Input: part model. Units: mm. Frame: model coordinates. Face numbers are marked on the shaded views. Coordinates: 2 decimals unless noted, no trailing zeros. Order: outer loops, then holes, each group sorted by start corner. A loop starts at its lowest first (then second) coordinate and runs counter-clockwise, first axis right, second up. Notation, with made-up numbers: (38, -7.75) -> (54, -7.75) arc R23 ccw to (54, 16.25) -> close; hole circle Ø1 at (-6.5, -9.75). An arc over 180 degrees is marked (long way). Answer as CSV lines item,"result".
from build123d import *

# Parameters (mm, degrees)
F0_R     = 507.5
F0_R_2   = 16.5
F0_R_3   = 410
F1_DEPTH = 56


with BuildPart() as f1:
    # F0 (on Top) → F1 (new body)
    with BuildSketch(Plane.XY):
        Circle(F0_R)
        with Locations((-335.875721, -335.875721)):
            Circle(F0_R_2, mode=Mode.SUBTRACT)
        with Locations((-237.5, -411.362067)):
            Circle(F0_R_2, mode=Mode.SUBTRACT)
        with Locations((-122.939046, -458.814767)):
            Circle(F0_R_2, mode=Mode.SUBTRACT)
        with Locations((0, -475)):
            Circle(F0_R_2, mode=Mode.SUBTRACT)
        with Locations((-411.362067, -237.5)):
            Circle(F0_R_2, mode=Mode.SUBTRACT)
        with Locations((-458.814767, -122.939046)):
            Circle(F0_R_2, mode=Mode.SUBTRACT)
        with Locations((-475, 0)):
            Circle(F0_R_2, mode=Mode.SUBTRACT)
        Circle(F0_R_3, mode=Mode.SUBTRACT)
        with Locations((122.939046, -458.814767)):
            Circle(F0_R_2, mode=Mode.SUBTRACT)
        with Locations((237.5, -411.362067)):
            Circle(F0_R_2, mode=Mode.SUBTRACT)
        with Locations((335.875721, -335.875721)):
            Circle(F0_R_2, mode=Mode.SUBTRACT)
        with Locations((411.362067, -237.5)):
            Circle(F0_R_2, mode=Mode.SUBTRACT)
        with Locations((458.814767, -122.939046)):
            Circle(F0_R_2, mode=Mode.SUBTRACT)
        with Locations((475, 0)):
            Circle(F0_R_2, mode=Mode.SUBTRACT)
        with Locations((-458.814767, 122.939046)):
            Circle(F0_R_2, mode=Mode.SUBTRACT)
        with Locations((-411.362067, 237.5)):
            Circle(F0_R_2, mode=Mode.SUBTRACT)
        with Locations((-335.875721, 335.875721)):
            Circle(F0_R_2, mode=Mode.SUBTRACT)
        with Locations((-237.5, 411.362067)):
            Circle(F0_R_2, mode=Mode.SUBTRACT)
        with Locations((-122.939046, 458.814767)):
            Circle(F0_R_2, mode=Mode.SUBTRACT)
        with Locations((0, 475)):
            Circle(F0_R_2, mode=Mode.SUBTRACT)
        with Locations((458.814767, 122.939046)):
            Circle(F0_R_2, mode=Mode.SUBTRACT)
        with Locations((411.362067, 237.5)):
            Circle(F0_R_2, mode=Mode.SUBTRACT)
        with Locations((122.939046, 458.814767)):
            Circle(F0_R_2, mode=Mode.SUBTRACT)
        with Locations((237.5, 411.362067)):
            Circle(F0_R_2, mode=Mode.SUBTRACT)
        with Locations((335.875721, 335.875721)):
            Circle(F0_R_2, mode=Mode.SUBTRACT)
    extrude(amount=F1_DEPTH)


solid = f1.part
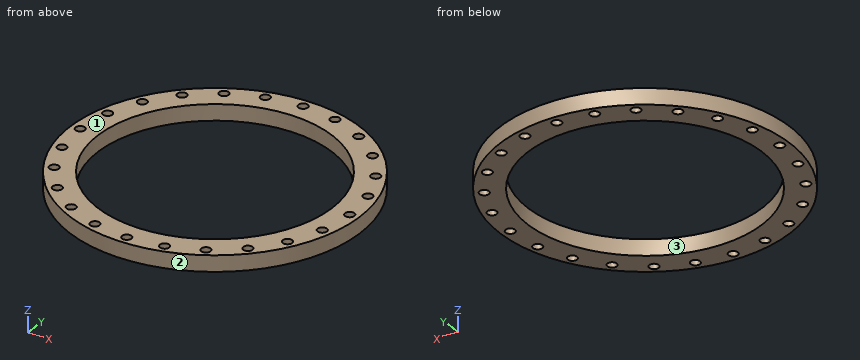
1. Cut plane A-A (y = 0). Return the cut outline in (x, z), plus the area to 3 significant figures.
Findings:
outline,"(-507.5, 0) -> (-491.5, 0) -> (-491.5, 56) -> (-507.5, 56) -> close; (-458.5, 0) -> (-410, 0) -> (-410, 56) -> (-458.5, 56) -> close; (410, 0) -> (458.5, 0) -> (458.5, 56) -> (410, 56) -> close; (491.5, 0) -> (507.5, 0) -> (507.5, 56) -> (491.5, 56) -> close"
area,"7,220 mm2"
2. Cut plane D-D (x = -84). Return the cut outline in (y, z), plus the area to 3 significant figures.
Findings:
outline,"(-500.5, 0) -> (-401.3, 0) -> (-401.3, 56) -> (-500.5, 56) -> close; (401.3, 0) -> (500.5, 0) -> (500.5, 56) -> (401.3, 56) -> close"
area,"11,100 mm2"
3. Ray query, line 1 along Y through (x, z) = (237.5, 40.5); line 2 along X through (y, z) = (13, 24); line 3 along X through (y, z) = (-4.5, 51.5). Return the intervals inside material, ascending.
Findings:
line 1,"y = -448.5 to -427.86, -394.86 to -334.21, 334.21 to 394.86, 427.86 to 448.5"
line 2,"x = -507.33 to -485.16, -464.84 to -409.79, 409.79 to 464.84, 485.16 to 507.33"
line 3,"x = -507.48 to -490.87, -459.13 to -409.98, 409.98 to 459.13, 490.87 to 507.48"
4. Cut plane C-C (y = 373.5). Return the cut outline in (x, z).
Findings:
outline,"(-343.59, 0) -> (-169.11, 0) -> (-169.11, 56) -> (-343.59, 56) -> close; (169.11, 0) -> (343.59, 0) -> (343.59, 56) -> (169.11, 56) -> close"
5. Contact query for flat-ended pins moving along their axis: pin 1 (20 mm diameter, centred on x = -411.36, y = 237.5, fed in from +Z); pin 2 (12 mm diameter, centred on x = 90.5, z = 14.5, fed in from -Y); pin 3 (4 mm diameter, centred on y = -223.5, z = 21, fed in from +X); pin 4 (12 mm diameter, centred on x = 152.5, z = 31.5, fed in from -Y). Output: stop coordinate, or through.
Findings:
pin 1,"passes through"
pin 2,"stops at y = -500.42"
pin 3,"stops at x = 456.61"
pin 4,"stops at y = -485.9"
6. Cut plane B-B (x = -237.5). Return the cut outline in (y, z), plus the area to 3 significant figures.
Findings:
outline,"(-448.5, 0) -> (-427.86, 0) -> (-427.86, 56) -> (-448.5, 56) -> close; (-394.86, 0) -> (-334.21, 0) -> (-334.21, 56) -> (-394.86, 56) -> close; (334.21, 0) -> (394.86, 0) -> (394.86, 56) -> (334.21, 56) -> close; (427.86, 0) -> (448.5, 0) -> (448.5, 56) -> (427.86, 56) -> close"
area,"9,100 mm2"
7. Mould query, pull axis X, two halves, no side actions, for the marked faces 1, 2 and 3. Classes: released by +X, released by -X, zero draft, split by the parting line, or undercut.
Findings:
face 1,"zero draft"
face 2,"split by the parting line"
face 3,"undercut"
